Geometry check sheet. Reference: the model listing, model coordinates, mm. A direction names the side the tool comes from. Coordinates: 2 decimals unless noted, no trailing zeros. Write each loop counter-clockwise with the first axis right and the second up, starting at its lowest first coordinate (ties: lowest second). Pieces come first, ordered by that corner, then holes. Notation, with made-up numbers: M -30,31.5 L 23,31.5 A12 ccw 23,46.5 Z; hole C 51,-6.75 d4. An arc over 180 degrees is marked long. Answer as a JSON object with one key per item and string values. Group by question number.
Autodesk Inventor part; units mm, degrees
ref_plane "Work Plane2" through (0, 0, 10) normal (0, 0, 1) x (1, 0, 0)
ref_plane "Work Plane8" through (0, 0, 0) normal (0.9238795, 0.3826834, 0) x (0, 0, 1)
ref_plane "Work Plane9" through (0, 0, 0) normal (1, 0, 0) x (0, 1, 0)
sketch "Sketch1" plane through (0, 0, 0) normal (0, 0, 1) x (1, 0, 0)
  circle A0 centre (0, 0) radius 6.25
  dimension "d0" = 12.5
extrude "Extrusion1" add sketch "Sketch1" along normal blind 20
ref_plane "Work Plane2" through (0, 0, 10) normal (0, 0, 1) x (1, 0, 0)
sketch "Sketch2" plane through (0, 0, 0) normal (0, 0, -1) x (-1, 0, 0)
  circle A0 centre (0, 0) radius 6.25
  circle A1 centre (0, 0) radius 5
  dimension "d3" = 10
surface extrude "Pitch Diameter" sketch "Sketch2" against normal through all shown no curves A1
ref_plane "Work Plane8" through (0, 0, 0) normal (0.9238795, 0.3826834, 0) x (0, 0, 1)
ref_plane "Work Plane9" through (0, 0, 0) normal (1, 0, 0) x (0, 1, 0)
spur gear teeth "Spur Gear" teeth 8 pitch diameter 10 tip diameter 12.5 root diameter 6.875 face width 20 start plane through (0, 0, 0) normal (0, 0, -1) x (-1, 0, 0)
equation "\"d0\" = da_da"
equation "\"d1\" = da_b"
equation "\"d3\" = da_d"
properties part number "Spur Gear1" material "Steel"
1) Draft check along Y on faces 1 (the cylindrical face through (0.01, -6.25, 9.86)), 2 (the cylindrical face through (4.1, 2.7, 9.9)), 3 (the cylindrical face through (4.41, 4.43, 9.86)). Enter one of: +Y half, -Y half, draft (parallel to the pull), parting line (faces both ways), or undercut.
2) Section check C-C (x = 5.75). Record the cut outline in (y, z), then the cut area to 3 significant figures.
3) Section check B-B (y = -2.5). Record the cut outline in (x, z).
4) Go/stop test with flat-tipped pins: pin 1 Ø6 at (x, y) = (4.5, 3) entering from -Z; pin 2 Ø3 at (x, z) = (-2, 10.5) entering from +Y. Record where each tip stops, or that it passes through.
5) Material ranges on probe 1 along Y at (x, z) = (-4.75, 2); probe 2 along Y at (x, z) = (3.75, 2.5); probe 3 along X at (y, z) = (-4, 19), recorded low to high. Write a range as [from, to].
6) Set-up check for faces 4 (the cylindrical face through (-2.7, -4.1, 9.9)), 5 (the cylindrical face through (4.1, -2.7, 9.9)), 6 (the cylindrical face through (2.7, 4.1, 9.9)), 7 (the cylindrical face through (0.996, -4.759, 9.86)): record each of +Z, -Z, +X, -X, +Y, -Y from which the full face is reachable in a straight line by a thin tool's end or side.
Entries:
{
 "1": {"face 1": "-Y half", "face 2": "undercut", "face 3": "+Y half"},
 "2": {"outline": "M -0.78,0 L 0.78,0 L 0.78,20 L -0.78,20 Z", "area": "31.2 mm^2"},
 "3": {"outline": "M -3.94,0 L 3.94,0 L 3.94,20 L -3.94,20 Z"},
 "4": {"pin 1": "z = 0", "pin 2": "y = 6.23"},
 "5": {"probe 1": "[-4.06, -3.78], [-1, 1], [3.78, 4.06]", "probe 2": "[-4.74, -2.28], [-1.04, 1.04], [2.28, 4.74]", "probe 3": "[-4.8, -2.57], [-1.04, 1.04], [2.57, 4.8]"},
 "6": {"face 4": "+Z, -Z, -Y", "face 5": "+Z, -Z, +X", "face 6": "+Z, -Z, +Y", "face 7": "+Z, -Z"}
}
